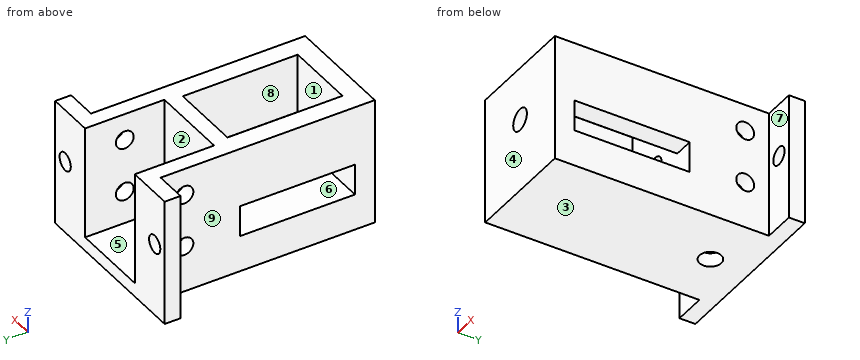
```python
from build123d import *

# Parameters (mm, degrees)
BOSS_EXTRUDE1_DEPTH = 27
SKETCH2_R           = 2.25
CUT_EXTRUDE1_DEPTH  = 52
SKETCH3_R           = 2.25
CUT_EXTRUDE2_DEPTH  = 41.162171256
SKETCH5_W           = 28
SKETCH5_H           = 4.176671075
BOSS_EXTRUDE2_DEPTH = 34
SKETCH6_W           = 28
SKETCH6_H           = 5
BOSS_EXTRUDE3_DEPTH = 22.823328925
SKETCH7_R           = 2.75
CUT_EXTRUDE3_DEPTH  = 68.653529103
BOSS_EXTRUDE4_REACH = 50.672
SKETCH8_W           = 5
SKETCH8_H           = 15
SKETCH9_R           = 2.75
BOSS_EXTRUDE5_DEPTH = 5
SKETCH10_W          = 20
SKETCH10_H          = 20
CUT_EXTRUDE4_DEPTH  = 1.5


with BuildPart() as part:
    # Sketch1 → Boss-Extrude1 (new body)
    with BuildSketch(Plane.XY):
        Polygon((-14, 0), (14, 0), (14, 20), (22, 20), (22, 24), (10, 24), (10, 4), (-10, 4), (-10, 24), (-22, 24), (-22, 20), (-14, 20), align=None)
    extrude(amount=BOSS_EXTRUDE1_DEPTH)

    # Sketch2 → Cut-Extrude1 (cut, through all)
    with BuildSketch(Plane.ZY.offset(14)):
        with Locations(Location((6.75, 14, 0), (0, 0, 270))):
            Circle(SKETCH2_R)
        with Locations(Location((20.25, 14, 0), (0, 0, 270))):
            Circle(SKETCH2_R)
    extrude(amount=-CUT_EXTRUDE1_DEPTH, mode=Mode.SUBTRACT)

    # Sketch3 → Cut-Extrude2 (cut, through all)
    with BuildSketch(Plane.XZ.offset(-20)):
        with Locations(Location((-18, 13.5, 0), (0, 0, 270))):
            Circle(SKETCH3_R)
        with Locations(Location((18, 13.5, 0), (0, 0, 270))):
            Circle(SKETCH3_R)
    extrude(amount=-CUT_EXTRUDE2_DEPTH, mode=Mode.SUBTRACT)

    # Sketch5 → Boss-Extrude2 (add)
    with BuildSketch(Plane.XZ):
        with Locations((0, 2.088335538)):
            Rectangle(SKETCH5_W, SKETCH5_H)
    extrude(amount=BOSS_EXTRUDE2_DEPTH)

    # Sketch6 → Boss-Extrude3 (add)
    with BuildSketch(Plane.XY.offset(4.176671075)):
        with Locations((0, -31.5)):
            Rectangle(SKETCH6_W, SKETCH6_H)
    extrude(amount=BOSS_EXTRUDE3_DEPTH)

    # Sketch7 → Cut-Extrude3 (cut, through all)
    with BuildSketch(Plane.XZ.offset(34)):
        with Locations(Location((0, 13.5, 0), (0, 0, 270))):
            Circle(SKETCH7_R)
    extrude(amount=-CUT_EXTRUDE3_DEPTH, mode=Mode.SUBTRACT)

    # Sketch8 → Boss-Extrude4 (add, up to next)
    with BuildSketch(Plane.XZ, mode=Mode.PRIVATE) as boss_extrude4_sk1:
        with Locations((11.5, 19.5)):
            Rectangle(SKETCH8_W, SKETCH8_H)
    boss_extrude4_tool1 = extrude(boss_extrude4_sk1.sketch, amount=BOSS_EXTRUDE4_REACH, mode=Mode.PRIVATE) - part.part
    # Sketch8 → Boss-Extrude4 (add, up to next)
    with BuildSketch(Plane.XZ, mode=Mode.PRIVATE) as boss_extrude4_sk2:
        with Locations((-11.5, 19.5)):
            Rectangle(SKETCH8_W, SKETCH8_H)
    boss_extrude4_tool2 = extrude(boss_extrude4_sk2.sketch, amount=BOSS_EXTRUDE4_REACH, mode=Mode.PRIVATE) - part.part
    add(boss_extrude4_tool1.solids().sort_by_distance((11.5, 0, 19.5))[0])
    add(boss_extrude4_tool2.solids().sort_by_distance((-11.5, 0, 19.5))[0])

    # Sketch9 → Boss-Extrude5 (add)
    with BuildSketch(Plane(origin=(0, 0, 0), x_dir=(-1, 0, 0), z_dir=(0, 0, -1))):
        Polygon((-14, -34), (14, -34), (14, 20), (22, 20), (22, 24), (-22, 24), (-22, 20), (-14, 20), align=None)
        with Locations((0, 14)):
            Circle(SKETCH9_R, mode=Mode.SUBTRACT)
    extrude(amount=BOSS_EXTRUDE5_DEPTH)

    # Sketch10 → Cut-Extrude4 (cut)
    with BuildSketch(Plane.XY):
        with Locations((0, 14)):
            Rectangle(SKETCH10_W, SKETCH10_H)
    extrude(amount=-CUT_EXTRUDE4_DEPTH, mode=Mode.SUBTRACT)


solid = part.part
```
The model under review builds one solid part; all positions refer to its coordinate system, in mm. Face numbers are marked on the shaded views. A direction names the side the tool comes from. Give positions to 0.01 mm unless a question says otherwise; leave off trailing zeros. Loops run counter-clockwise (first coordinate to the right, second up) from the corner with the lowest first, then second, coordinate; pieces in that order, holes last. Notation, with made-up numbers: (48, 65) -> (60, 65) arc R15 ccw to (60, 73) -> close; hole circle Ø1 at (-7, 10.25). An arc over 180 degrees is marked (long way). Use CSV: the item, a comma, the result in double quotes.
1. Consider section A-A, the plane z = 20.25. Write out the cut boundary in (x, y), then the cut area to 3 significant figures.
Result:
outline,"(-22, 20) -> (-14, 20) -> (-14, 16.25) -> (-10, 16.25) -> (-10, 24) -> (-22, 24) -> close; (-14, -34) -> (14, -34) -> (14, 11.75) -> (10, 11.75) -> (10, 4) -> (-10, 4) -> (-10, 11.75) -> (-14, 11.75) -> close; (10, 16.25) -> (14, 16.25) -> (14, 20) -> (22, 20) -> (22, 24) -> (10, 24) -> close; hole (-9, -29) -> (9, -29) -> (9, 0) -> (-9, 0) -> close"
area,"730 mm²"
2. For P1, Ø2.5, axis at x = -17, z = 14, coming from the -Y side; P2, Ø1, axis at x = -2.5, y = -28, coming from the +Z side; P3, Ø16, axis at y = 9.5, z = 17, coming from the -X side; P4, Ø22, axis at x = 4.5, y = 10.5, coming from the +Z side, all flat-tipped, find the tip position at first contact; note any pin that passes through.
Result:
P1,"stops at y = 20"
P2,"stops at z = 4.18"
P3,"stops at x = -14"
P4,"stops at z = 27"
3. Machinability: for the marked faces 5, 6, 7, 8 and 9, which of the approach directions +Z, -Z, +X, -X, +Y, -Y give a long, thin tool a straight path to every point of the face, cutting with its end or side? Answer none if there is none.
Result:
face 5,"+Z, +Y"
face 6,"+X, -X"
face 7,"+Z, -Z, +X, -Y"
face 8,"+Z"
face 9,"+Z, -Z, -X, -Y"
4. Consider section D-D, the plane y = -21. Write out the cut boundary in (x, z), then the cut area to 3 significant figures.
Result:
outline,"(-14, -5) -> (14, -5) -> (14, 4.18) -> (-14, 4.18) -> close; (-14, 12) -> (-9, 12) -> (-9, 27) -> (-14, 27) -> close; (9, 12) -> (14, 12) -> (14, 27) -> (9, 27) -> close"
area,"407 mm²"
5. The part is to be moulded in two halves that separate along Y. For the marked faces 1, 2, 3 and 4, say which applies: +Y half, -Y half, draft (parallel to the pull), parting line (faces both ways), or undercut.
Result:
face 1,"undercut"
face 2,"+Y half"
face 3,"draft"
face 4,"-Y half"
6. To check wall thickness, follow probe 1 along X at (y, z) = (22.7, 13.5); probe 2 along X at (y, z) = (-6, 24); probe 3 along Y at (x, z) = (4, 20.5). State the ranges of each line that lie inside material, in increasing order. Write a range as from..to.
Result:
probe 1,"x = -22..-20.25, -15.75..-10, 10..15.75, 20.25..22"
probe 2,"x = -14..-9, 9..14"
probe 3,"y = -34..-29, 0..4"
7. Consider section C-C, the plane x = -18. Write out the cut boundary in (y, z).
Result:
outline,"(20, -5) -> (24, -5) -> (24, 11.25) -> (20, 11.25) -> close; (20, 15.75) -> (24, 15.75) -> (24, 27) -> (20, 27) -> close"
8. Consider section B-B, the plane y = 14. Write out the cut boundary in (x, z), then the cut area to 3 significant figures.
Result:
outline,"(-14, -5) -> (-2.75, -5) -> (-2.75, -1.5) -> (-10, -1.5) -> (-10, 4.5) -> (-14, 4.5) -> close; (-14, 9) -> (-10, 9) -> (-10, 18) -> (-14, 18) -> close; (-14, 22.5) -> (-10, 22.5) -> (-10, 27) -> (-14, 27) -> close; (2.75, -5) -> (14, -5) -> (14, 4.5) -> (10, 4.5) -> (10, -1.5) -> (2.75, -1.5) -> close; (10, 9) -> (14, 9) -> (14, 18) -> (10, 18) -> close; (10, 22.5) -> (14, 22.5) -> (14, 27) -> (10, 27) -> close"
area,"235 mm²"
